Model file for the job. Use its own axes, mm. A direction names the side the tool comes from. Give positions to 0.01 mm unless a question says otherwise; leave off trailing zeros. Loops run counter-clockwise (first coordinate to the right, second up) from the corner with the lowest first, then second, coordinate; pieces in that order, holes last. Notation, with made-up numbers: (56.5, 75.5) - (93.5, 75.5) arc R11 ccw to (93.5, 92.5) - close; hole circle Ø6 at (78, -14). An arc over 180 degrees is marked (long way). Use a Markdown table: item, result.
from build123d import *

# Parameters (mm, degrees)
F1_DEPTH = 19.05
F2_W     = 19.05
F2_H     = 19.05
F3_DEPTH = 19.05
F4_W     = 19.05
F4_H     = 38.1
F5_DEPTH = 6.35


with BuildPart() as f1:
    # F0 (on Top) → F1 (new body)
    with BuildSketch(Plane.XY):
        Polygon((47.625, 222.31108), (-47.625, 222.31108), (-216.339543, -69.91108), (-168.714543, -152.4), (168.714543, -152.4), (216.339543, -69.91108), align=None)
    extrude(amount=F1_DEPTH)

    # F2 (on face) → F3 (cut, through all)
    with BuildSketch(Plane.XY.offset(19.05)):
        with Locations((0, 174.68608)):
            Rectangle(F2_W, F2_H)
        Polygon((154.768975, -100.354432), (164.293975, -83.856648), (147.796191, -74.331648), (138.271191, -90.829432), align=None)
        Polygon((-164.293975, -83.856648), (-154.768975, -100.354432), (-138.271191, -90.829432), (-147.796191, -74.331648), align=None)
    extrude(amount=-F3_DEPTH, mode=Mode.SUBTRACT)

    # F4 (on face) → F5 (cut)
    with BuildSketch(Plane.XY.offset(19.05)):
        Polygon((-154.768975, -100.354432), (-164.293975, -83.856648), (-197.289543, -102.906648), (-187.764543, -119.404432), align=None)
        Polygon((197.289543, -102.906648), (164.293975, -83.856648), (154.768975, -100.354432), (187.764543, -119.404432), align=None)
        with Locations((0, 203.26108)):
            Rectangle(F4_W, F4_H)
    extrude(amount=-F5_DEPTH, mode=Mode.SUBTRACT)


solid = f1.part
(1) Pin check, flat tips, straight feed: P1, Ø5, axis at y = -32.5, z = 2.5, coming from the -X side; P2, Ø3, axis at y = 0.5, z = 11, coming from the -X side; P3, Ø1, axis at y = 75.5, z = 13.5, coming from the +X side. Stop position of each tip, or through.
Computed:
| item | result |
|---|---|
| P1 | x = -196.18 |
| P2 | x = -176.55 |
| P3 | x = 132.68 |
(2) Slice it at D-D, the plane x = -101. Write the cut outline in (y, z), plus the area to 3 significant figures.
Computed:
| item | result |
|---|---|
| outline | (-152.4, 0) - (129.86, 0) - (129.86, 19.05) - (-152.4, 19.05) - close |
| area | 5,380 mm² |
(3) Mould opens along Y. For faces 1 (the flat face through (133.163, 74.154, 9.392)), 2 (the flat face through (0, 204, 12.7)), 3 (the flat face through (159.465, -92.221, 6.439)), 4 (the flat face through (-192.86, -110.58, 9.39)) say: pulls with the +Y half, pulls with the -Y half, needs draft (parallel to the pull), parting line crosses it, or undercut.
Computed:
| item | result |
|---|---|
| face 1 | pulls with the +Y half |
| face 2 | needs draft |
| face 3 | undercut |
| face 4 | pulls with the -Y half |
(4) Slice it at A-A, the plane y = 177. Write the cut outline in (x, z) (3 decimals), plus the area to 3 significant figures.
Computed:
| item | result |
|---|---|
| outline | (-73.785, 0) - (-9.525, 0) - (-9.525, 19.05) - (-73.785, 19.05) - close; (9.525, 0) - (73.785, 0) - (73.785, 19.05) - (9.525, 19.05) - close |
| area | 2,450 mm² |
(5) Slice it at B-B, the plane z = 16. Write the cut outline in (x, y) (3 decimals).
Computed:
| item | result |
|---|---|
| outline | (-216.34, -69.911) - (-197.29, -102.907) - (-147.796, -74.332) - (-138.271, -90.829) - (-187.765, -119.404) - (-168.715, -152.4) - (168.715, -152.4) - (187.765, -119.404) - (138.271, -90.829) - (147.796, -74.332) - (197.29, -102.907) - (216.34, -69.911) - (47.625, 222.311) - (9.525, 222.311) - (9.525, 165.161) - (-9.525, 165.161) - (-9.525, 222.311) - (-47.625, 222.311) - close |
(6) Drill centre lines: probe 1 along X at (y, z) = (-84, 14.75); probe 2 along X at (y, z) = (-84.5, 13.5); probe 3 along Y at (x, z) = (-8, 14). Where is each one in solid material? Low to high. Write a range as [from, to].
Computed:
| item | result |
|---|---|
| probe 1 | [-208.21, -164.54], [-142.21, 142.21], [164.54, 208.21] |
| probe 2 | [-207.92, -165.41], [-141.93, 141.93], [165.41, 207.92] |
| probe 3 | [-152.4, 165.16] |
(7) 3-axis set-ups, long thin cutter, end or side, ignore diameter. For faces 5 (the flat face through (192.194, -111.733, 9.392)), 6 (the flat face through (0, 165.161, 10)), 7 (the flat face through (-157.865, -102.142, 13.892)): which of +Z, -Z, +X, -X, +Y, -Y reach the whole face in a straight line?
Computed:
| item | result |
|---|---|
| face 5 | +Z, -Z, +X, -Y |
| face 6 | +Z, -Z |
| face 7 | +Z |
(8) Slice it at C-C, the plane y = -112.5. Write the cut outline in (x, z), plus the area to 3 significant figures.
Computed:
| item | result |
|---|---|
| outline | (-191.75, 0) - (191.75, 0) - (191.75, 12.7) - (175.81, 12.7) - (175.81, 19.05) - (-175.81, 19.05) - (-175.81, 12.7) - (-191.75, 12.7) - close |
| area | 7,100 mm² |
